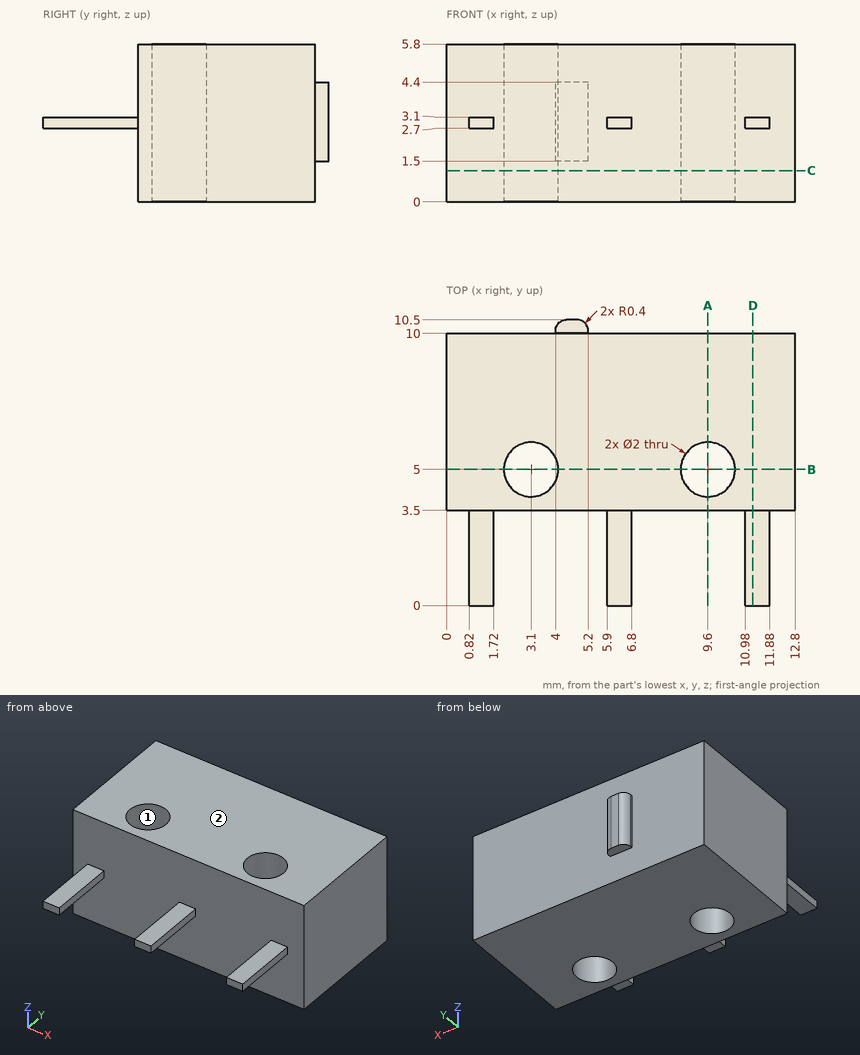
Geometry: see drawing. Coordinates: mm, zero at the bounding-box minimum. Give positions to 0.01 mm unless a question says otherwise; leave off trailing zeros. Loops run counter-clockwise (first coordinate to the right, second up) from the corner with the lowest first, then second, coordinate; pieces in that order, holes last. Notation, with made-up numbers: (76, 14) - (114, 14) arc R22 ccw to (114, 37) - close; hole circle Ø7 at (-2.5, 68). An arc over 180 degrees is marked (long way). Use CSV: the item, a comma, the result in double quotes. Start each with the question number.
Item 1: Section C-C on z = 1.15. Return loops of the section in (x, y).
Item 2: Line query: line 1 (Y direction, x = 9.6, z = 3.8); line 2 (Y direction, x = 2, z = 1.1); line 3 (Y direction, x = 4.5, z = 1.7). Output: solid intervals per line, ascending.
Item 3: Section D-D on x = 11.25. Return loops of the section in (y, z).
Item 4: Section B-B on y = 5. Return loops of the section in (x, z), then the cut area to 3 significant figures.
Item 5: Mould query, pull axis Y, two halves, no side actions, for the marked faces 1 and 2. Classes: pulls with the +Y half, pulls with the -Y half, needs draft (parallel to the pull), parting line crosses it, or undercut.
Item 6: Section A-A on x = 9.6. Return loops of the section in (y, z).
Item 7: Contact query for flat-ended pins moving along their axis: P1, Ø3, axis at x = 8, z = 2.5, coming from the +Y side; P2, Ø1, axis at x = 1, y = 1.5, coming from the +Z side; P3, Ø1.8, axis at x = 3.1, y = 5, coming from the -Z side; P4, Ø0.5, axis at x = 11, y = 2.5, coming from the -Z side. Output: stop coordinate, or through.
Ans:
1,outline,"(0, 3.5) - (12.8, 3.5) - (12.8, 10) - (0, 10) - close; hole circle Ø2 at (3.1, 5); hole circle Ø2 at (9.6, 5)"
2,line 1,"y = 3.5 to 4, 6 to 10"
2,line 2,"y = 3.5 to 10"
2,line 3,"y = 3.5 to 10.5"
3,outline,"(0, 2.7) - (3.5, 2.7) - (3.5, 0) - (10, 0) - (10, 5.8) - (3.5, 5.8) - (3.5, 3.1) - (0, 3.1) - close"
4,outline,"(0, 0) - (2.1, 0) - (2.1, 5.8) - (0, 5.8) - close; (4.1, 0) - (8.6, 0) - (8.6, 5.8) - (4.1, 5.8) - close; (10.6, 0) - (12.8, 0) - (12.8, 5.8) - (10.6, 5.8) - close"
4,area,"51.0 mm2"
5,face 1,"undercut"
5,face 2,"needs draft"
6,outline,"(3.5, 0) - (4, 0) - (4, 5.8) - (3.5, 5.8) - close; (6, 0) - (10, 0) - (10, 5.8) - (6, 5.8) - close"
7,P1,"stops at y = 10"
7,P2,"stops at z = 3.1"
7,P3,"passes through"
7,P4,"stops at z = 2.7"
